Geometry check sheet. Reference: the model listing, model coordinates, mm. A direction names the side the tool comes from. Round coordinates to 2 decimals unless told otherwise and drop trailing zeros. Write each loop counter-clockwise with the first axis right and the second up, starting at its lowest first coordinate (ties: lowest second). Pieces come first, ordered by that corner, then holes. Notation, with made-up numbers: (3, -1.5) -> (14, -1.5) arc R9 cw to (14, 5.5) -> close; hole circle Ø5 at (-11.5, 25.5). An arc over 180 degrees is marked (long way). Use a Markdown table: item, result.
```python
from build123d import *

# Parameters (mm, degrees)
FILLET1_R                = 2
SKETCH5_R                = 8.5
SKETCH5_R_2              = 7
BOSS_EXTRUDE1_DEPTH      = 0.1
BOSS_EXTRUDE2_DEPTH      = 0.5
BOSS_EXTRUDE2_DEPTH_BACK = 0.5
SKETCH6_R                = 2
SKETCH6_R_2              = 1.5


with BuildPart() as part:
    # Sketch4 → Revolve1 (revolve)
    with BuildSketch(Plane(origin=(0, 0, 0), x_dir=(0, 0, -1), z_dir=(1, 0, 0))):
        Polygon((0, 0), (-3.75, 0), (-4.25, -0.5), (-4.75, 0), (-8.5, 0), (-8.5, -4), (0, -4), align=None)
    revolve(axis=Axis((0, 1.890471386, 0), (0, -1, 0)))

    # Fillet1
    fillet1_edges = [part.edges().sort_by_distance(p)[0] for p in [
        (0, 0, -8.5),
    ]]
    fillet(fillet1_edges, radius=FILLET1_R)



with BuildPart() as body_2:
    # Sketch5 → Boss-Extrude1 (new body)
    with BuildSketch(Plane.XZ.offset(4)):
        with Locations(Location((0, 0, 0), (0, 0, 90))):
            Circle(SKETCH5_R)
        with Locations(Location((0, 0, 0), (0, 0, 270))):
            Circle(SKETCH5_R_2, mode=Mode.SUBTRACT)
    extrude(amount=BOSS_EXTRUDE1_DEPTH)


with BuildPart() as part_1:
    add(part.part)

    add(body_2.part)  # Boss-Extrude2 merges body 2
    # Sketch6 → Boss-Extrude2 (add, two sides: drawn at the far end of the back side and taken through both)
    # profile 1 of 2: a face of its own
    with BuildSketch(Plane(origin=(0, 0, 0), x_dir=(0, 0, -1), z_dir=(1, 0, 0)).offset(-BOSS_EXTRUDE2_DEPTH_BACK)):
        with BuildLine():
            Line((13.132863069, 0.320027848), (0, 0))
            Line((0, 0), (0, -0.907670556))
            Line((0, -0.907670556), (7.174444166, -0.907670556))
            Line((7.174444166, -0.907670556), (8.5, -4))
            Line((8.5, -4), (13.12184584, -1.999779955))
            Line((13.12184584, -1.999779955), (14.746442499, -4.961787965))
            ThreePointArc((14.746442499, -4.961787965), (14.953109522, -2.732273748), (17.098589091, -2.09167846))
            ThreePointArc((17.098589091, -2.09167846), (14.968839585, -1.127360353), (13.132863069, 0.320027848))
        make_face()
    # profile 2 of 2: a face of its own
    with BuildSketch(Plane(origin=(0, 0, 0), x_dir=(0, 0, -1), z_dir=(1, 0, 0)).offset(-BOSS_EXTRUDE2_DEPTH_BACK)):
        with Locations((16.5, -4)):
            Circle(SKETCH6_R)
        with Locations((16.5, -4)):
            Circle(SKETCH6_R_2, mode=Mode.SUBTRACT)
    extrude(amount=BOSS_EXTRUDE2_DEPTH + BOSS_EXTRUDE2_DEPTH_BACK)


solid = part_1.part
```
(1) Thickness scan on line 1 (X direction, y = -4.05, z = 0); line 2 (Z direction, x = 0, y = -3.95); line 3 (X direction, y = -2, z = -12.75). Record the ranges inside material, lowest first.
A:
| item | result |
|---|---|
| line 1 | x = -8.5 to -7, 7 to 8.5 |
| line 2 | z = -18.5 to -18, -15 to -14.19, -8.62 to 8.5 |
| line 3 | x = -0.5 to 0.5 |
(2) Section check D-D on z = -13.5. Record the cut outline in (x, y).
A:
| item | result |
|---|---|
| outline | (-0.5, -2.69) -> (0.5, -2.69) -> (0.5, -0.03) -> (-0.5, -0.03) -> close |
(3) Section check C-C on y = -1.5. Record the cut outline in (x, z).
A:
| item | result |
|---|---|
| outline | (-0.5, -15.64) -> (0.5, -15.64) -> (0.5, -8.42) arc R8.44 ccw (long way) to (-0.5, -8.42) -> close |
(4) Access from +Z, -Z, +X, -X, +Y, -Y to the whole of each face (thin tool, end or side, straight path). Record for faces 3 (the face through (-0.01, -5.31, -18.01)), 4 (the face through (-0.007, -3.014, -10.779)).
A:
| item | result |
|---|---|
| face 3 | +X, -X |
| face 4 | +X, -X, -Y |
(5) Section check A-A on y = -4.5. Record the cut outline in (x, z), plus the area to 3 significant figures.
A:
| item | result |
|---|---|
| outline | (-0.5, -18.44) -> (0.5, -18.44) -> (0.5, -17.91) -> (-0.5, -17.91) -> close; (-0.5, -15.09) -> (0.5, -15.09) -> (0.5, -14.49) -> (-0.5, -14.49) -> close |
| area | 1.11 mm2 |
(6) Gauge pin test, flat ends, axial feed: pin 1 Ø2.5 at (y, z) = (-4, -16.5) entering from -X; pin 2 Ø4 at (x, z) = (-1, -1) entering from -Y; pin 3 Ø6 at (x, z) = (-6.5, -8) entering from +Y; pin 4 Ø2 at (x, y) = (-4, -4) entering from +Z. Record the tip position at first contact, or that the pin passes through.
A:
| item | result |
|---|---|
| pin 1 | passes through |
| pin 2 | stops at y = -4 |
| pin 3 | stops at y = -0.17 |
| pin 4 | stops at z = 7.95 |
(7) Release check for a two-part mould opening along X. For faces 1 (the face through (0, -4, 0)), 2 (the face through (-0.007, -3.46, -13.923)) record: +X half, -X half, draft (parallel to the pull), parting line (faces both ways), or undercut.
A:
| item | result |
|---|---|
| face 1 | undercut |
| face 2 | draft |
(8) Section check B-B on z = -16.5. Record the cut outline in (x, y), plus the area to 3 significant figures.
A:
| item | result |
|---|---|
| outline | (-0.5, -6) -> (0.5, -6) -> (0.5, -5.5) -> (-0.5, -5.5) -> close; (-0.5, -2.5) -> (0.5, -2.5) -> (0.5, -1.88) -> (-0.5, -1.88) -> close |
| area | 1.12 mm2 |
